Geometry: see drawing. Coordinates: mm, zero at the bounding-box minimum. Coordinates: 2 decimals unless noted, no trailing zeros. Order: outer loops, then holes, each group sorted by start corner. A loop starts at its lowest first (then second) coordinate and runs counter-clockwise, first axis right, second up.
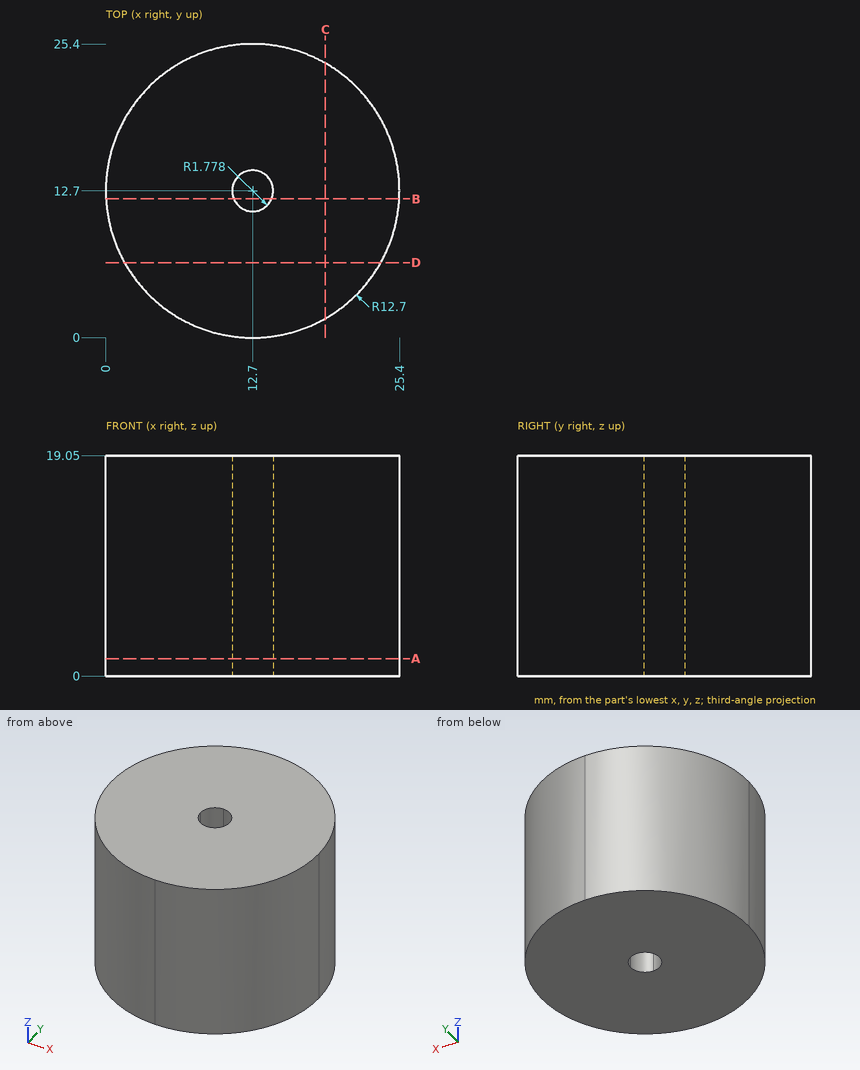
Q1. Section query D-D on y = 6.5. Output: boundary loops of the cut face in (x, z), plus the area to 3 significant figures.
Solutions:
outline: (1.62, 0) - (23.78, 0) - (23.78, 19.05) - (1.62, 19.05) - close
area: 422 mm2
Q2. Section query A-A on z = 1.5. Output: boundary loops of the cut face in (x, y), plus the area to 3 significant figures.
Solutions:
outline: circle Ø25.4 at (12.7, 12.7); hole circle Ø3.56 at (12.7, 12.7)
area: 497 mm2
Q3. Section query C-C on x = 19. Output: boundary loops of the cut face in (y, z).
Solutions:
outline: (1.67, 0) - (23.73, 0) - (23.73, 19.05) - (1.67, 19.05) - close
Q4. Pin query (flat end, axial travel): P1, Ø8, axis at y = 18, z = 9.5, coming from the +X side; P2, Ø6, axis at y = 5, z = 12, coming from the +X side; P3, Ø4, axis at x = 17.5, z = 2.5, coming from the +Y side. Return the tip coordinate at first contact, or that it passes through.
Solutions:
P1: stops at x = 25.33
P2: stops at x = 24.5
P3: stops at y = 25.09
Q5. Section query B-B on y = 12. Output: boundary loops of the cut face in (x, z), plus the area to 3 significant figures.
Solutions:
outline: (0.02, 0) - (11.07, 0) - (11.07, 19.05) - (0.02, 19.05) - close; (14.33, 0) - (25.38, 0) - (25.38, 19.05) - (14.33, 19.05) - close
area: 421 mm2
Q6. Material intervals for line 1 along Y through (x, z) = (24, 3.75); line 2 along Y through (x, z) = (7.25, 5.5); line 3 along X through (y, z) = (15, 11.5), sorted ascending.
Solutions:
line 1: y = 6.9 to 18.5
line 2: y = 1.23 to 24.17
line 3: x = 0.21 to 25.19
